Geometry: final body of the model. Coordinates: model frame, mm. Coordinates: 2 decimals unless noted, no trailing zeros. Order: outer loops, then holes, each group sorted by start corner. A loop starts at its lowest first (then second) coordinate and runs counter-clockwise, first axis right, second up. Notation, with made-up numbers: (-22, 60) -> (37, 60) arc R19 ccw to (37, 83) -> close; hole circle Ø3 at (72.5, -23.75). An arc over 180 degrees is marked (long way). Use one line per item in the form item = value.
Autodesk Inventor part; units mm, degrees
ref_plane "YZ Plane" through (0, 0, 0) normal (1, 0, 0) x (0, 1, 0)
ref_plane "XZ Plane" through (0, 0, 0) normal (0, 1, 0) x (-1, 0, 0)
ref_plane "XY Plane" through (0, 0, 0) normal (0, 0, 1) x (1, 0, 0)
sketch "Sketch1" plane through (0, 0, 0) normal (0, 0, 1) x (1, 0, 0)
  line L0 (0, 0) -> (50.8, 0) construction
  line L1 (50.8, 0) -> (50.8, 203.2) construction
  line L2 (50.8, 203.2) -> (0, 203.2) construction
  line L3 (0, 203.2) -> (0, 0) construction
  line L4 (-76.2, 0) -> (177.8, 0) construction
  line L5 (177.8, 0) -> (177.8, -76.2) construction
  line L6 (177.8, -76.2) -> (-76.2, -76.2) construction
  line L7 (-76.2, -76.2) -> (-76.2, 0) construction
  line L8 (165.1, -33.3375) -> (165.1, -68.2625) construction
  circle A0 centre (165.1, -33.3375) radius 4.7625 construction
  line L9 (174.625, -3.175) -> (-73.025, -3.175) construction
  line L10 (-73.025, -3.175) -> (-73.025, -73.025) construction
  line L11 (-73.025, -73.025) -> (174.625, -73.025) construction
  line L12 (174.625, -73.025) -> (174.625, -3.175) construction
  circle A1 centre (165.1, -68.2625) radius 4.7625 construction
  line L13 (-76.2, -76.2) -> (-76.2, 0)
  line L14 (-76.2, 0) -> (0, 101.6)
  line L15 (0, 101.6) -> (50.8, 101.6)
  line L16 (50.8, 101.6) -> (177.8, 0)
  line L17 (177.8, 0) -> (177.8, -76.2)
  line L18 (177.8, -76.2) -> (-76.2, -76.2)
  line L19 (50.8, 101.6) -> (50.8, 0) construction
  line L20 (50.8, 0) -> (177.8, 0) construction
  line L21 (0, 101.6) -> (0, 0) construction
  line L22 (0, 0) -> (-76.2, 0) construction
  line L23 (60.325, 9.525) -> (60.325, 77.7161) construction
  line L24 (50.8, 85.3361) -> (157.4701, 0)
  line L25 (145.5638, 9.525) -> (60.325, 9.525) construction
  line L26 (-60.325, 0) -> (0, 80.4333)
  line L27 (-9.525, 67.7333) -> (-9.525, 9.525) construction
  line L28 (-9.525, 9.525) -> (-53.1813, 9.525) construction
  line L29 (-60.325, 0) -> (0, 0)
  line L30 (0, 80.4333) -> (0, 0)
  line L31 (50.8, 85.3361) -> (50.8, 0)
  line L32 (50.8, 0) -> (157.4701, 0)
  line L33 (-9.525, 9.525) -> (-9.525, 0) construction
  line L34 (0, 4.7625) -> (50.8, 4.7625) construction
  line L35 (12.7, 34.925) -> (38.1, 34.925) construction
  line L36 (-6.35, 71.9667) -> (-6.35, 0)
  line L37 (57.15, 80.2561) -> (57.15, 0)
  point P0 (152.4, -50.8)
  point P1 (165.1, -50.8)
  point P2 (139.7, -68.2625)
  point P3 (139.7, -33.3375)
  point P4 (127, -50.8)
  point P5 (114.3, -68.2625)
  point P6 (114.3, -33.3375)
  point P7 (101.6, -50.8)
  point P8 (88.9, -68.2625)
  point P9 (88.9, -33.3375)
  point P10 (76.2, -50.8)
  point P11 (63.5, -68.2625)
  point P12 (63.5, -33.3375)
  point P13 (50.8, -50.8)
  point P14 (38.1, -68.2625)
  point P15 (38.1, -33.3375)
  point P16 (25.4, -50.8)
  point P17 (12.7, -68.2625)
  point P18 (12.7, -33.3375)
  point P19 (0, -50.8)
  point P20 (-12.7, -68.2625)
  point P21 (-12.7, -33.3375)
  point P22 (-25.4, -50.8)
  point P23 (-38.1, -68.2625)
  point P24 (-38.1, -33.3375)
  point P25 (-50.8, -50.8)
  point P26 (-63.5, -68.2625)
  point P27 (-63.5, -33.3375)
  point P28 (-76.2, -50.8)
  point P29 (12.7, 76.2)
  point P30 (38.1, 76.2)
  point P31 (-9.525, 4.7625)
  point P32 (25.4, 4.7625)
  point P33 (25.4, 34.925)
  dimension "d0" = 50.8
  dimension "d1" = 203.2
  dimension "d2" = 254
  dimension "d3" = 76.2
  dimension "d4" = 127
  dimension "d5" = 12.7
  dimension "d6" = 12.7
  dimension "d7" = 9.525
  dimension "d8" = 3.175
  dimension "d9" = 9.525
  dimension "d12" = 25.4
  dimension "d17" = 25.4
  dimension "d18" = 34.925
  dimension "d19" = 25.4
  dimension "d20" = 12.7
  dimension "d21" = 9.525
  dimension "d22" = 9.525
  dimension "d32" = 111.125
  dimension "d33" = 41.275
  dimension "d35" = 12.7
  dimension "d36" = 12.7
  dimension "d37" = 9.525
  dimension "d38" = 50.8
  dimension "d39" = 34.925
  dimension "d40" = 6.35
  dimension "d41" = 6.35
extrude "Extrusion1" add sketch "Sketch1" along normal blind 6.35 contours L13 L14 L15 L16 L17 L18 | L24 L37 L32 L31 | L26 L30 L29 L36
hole "Hole1" at (165.1, -33.3375, 0) at (165.1, -68.2625, 0) at (139.7, -68.2625, 0) at (139.7, -33.3375, 0) at (-38.1, -33.3375, 0) at (-63.5, -68.2625, 0) at (-63.5, -33.3375, 0) at (12.7, 76.2, 0) at (38.1, 76.2, 0) at (38.1, 34.925, 0) at (12.7, 34.925, 0) at (-38.1, -68.2625, 0) at (-12.7, -33.3375, 0) at (-12.7, -68.2625, 0) at (63.5, -33.3375, 0) at (63.5, -68.2625, 0) direction (0, 0, 1) diameter 3.9624 end through all
fillet "Fillet1" radius 6.604 12 edges at (50.8, 101.6, 3.175) (0, 101.6, 3.175) (177.8, 0, 3.175) (-76.2, 0, 3.175) (-76.2, -76.2, 3.175) (177.8, -76.2, 3.175) (-60.325, 0, 3.175) (157.4701, 0, 3.175) (-6.35, 0, 3.175) (57.15, 0, 3.175) (57.15, 80.2561, 3.175) (-6.35, 71.9667, 3.175)
sketch "Sketch2" plane through (0, 0, 6.35) normal (0, 0, 1) x (1, 0, 0)
  line L0 (0, -19.05) -> (50.8, -19.05)
  line L1 (50.8, -19.05) -> (50.8, -63.5)
  line L2 (50.8, -63.5) -> (0, -63.5)
  line L3 (0, -63.5) -> (0, -19.05)
  arc A0 (-6.35, 52.1547) -> (-18.2372, 56.1171) centre (-12.954, 52.1547) ccw
  line L4 (-18.2372, 56.1171) -> (-52.4002, 10.5664)
  arc A1 (-52.4002, 10.5664) -> (-47.117, 0) centre (-47.117, 6.604) ccw
  line L5 (-47.117, 0) -> (-12.954, 0)
  arc A2 (-12.954, 0) -> (-6.35, 6.604) centre (-12.954, 6.604) ccw
  line L6 (-6.35, 6.604) -> (-6.35, 52.1547)
  arc A3 (57.15, 6.604) -> (63.754, 0) centre (63.754, 6.604) ccw
  line L7 (63.754, 0) -> (138.6435, 0)
  arc A4 (138.6435, 0) -> (142.769, 11.7609) centre (138.6435, 6.604) ccw
  line L8 (142.769, 11.7609) -> (67.8795, 71.6725)
  arc A5 (67.8795, 71.6725) -> (57.15, 66.5156) centre (63.754, 66.5156) ccw
  line L9 (57.15, 66.5156) -> (57.15, 6.604)
  arc A6 (3.302, 101.6) -> (-1.9812, 98.9584) centre (3.302, 94.996) ccw
  line L10 (3.302, 101.6) -> (48.4834, 101.6)
  arc A7 (52.6089, 100.1529) -> (48.4834, 101.6) centre (48.4834, 94.996) ccw
  line L11 (52.6089, 100.1529) -> (175.3215, 1.9828)
  arc A8 (177.8, -3.174) -> (175.3215, 1.9828) centre (171.196, -3.174) ccw
  line L12 (177.8, -3.174) -> (177.8, -69.596)
  arc A9 (171.196, -76.2) -> (177.8, -69.596) centre (171.196, -69.596) ccw
  line L13 (171.196, -76.2) -> (-69.596, -76.2)
  arc A10 (-76.2, -69.596) -> (-69.596, -76.2) centre (-69.596, -69.596) ccw
  line L14 (-76.2, -69.596) -> (-76.2, -2.2013)
  arc A11 (-74.8792, 1.7611) -> (-76.2, -2.2013) centre (-69.596, -2.2013) ccw
  line L15 (-74.8792, 1.7611) -> (-1.9812, 98.9584)
  circle A12 centre (12.7, 34.925) radius 1.9812
  circle A13 centre (38.1, 76.2) radius 1.9812
  circle A14 centre (-63.5, -33.3375) radius 1.9812
  circle A15 centre (-38.1, -33.3375) radius 1.9812
  circle A16 centre (139.7, -68.2625) radius 1.9812
  circle A17 centre (165.1, -33.3375) radius 1.9812
  circle A18 centre (165.1, -68.2625) radius 1.9812
  circle A19 centre (139.7, -33.3375) radius 1.9812
  circle A20 centre (-63.5, -68.2625) radius 1.9812
  circle A21 centre (12.7, 76.2) radius 1.9812
  circle A22 centre (38.1, 34.925) radius 1.9812
  circle A23 centre (-38.1, -68.2625) radius 1.9812
  circle A24 centre (-12.7, -68.2625) radius 1.9812
  circle A25 centre (-12.7, -33.3375) radius 1.9812
  line L16 (76.2, -19.05) -> (127, -19.05)
  line L17 (127, -19.05) -> (127, -63.5)
  line L18 (127, -63.5) -> (76.2, -63.5)
  line L19 (76.2, -63.5) -> (76.2, -19.05)
  circle A26 centre (63.5, -33.3375) radius 1.9812
  circle A27 centre (63.5, -68.2625) radius 1.9812
  point P0 (0, 0)
  dimension "d44" = 12.7
  dimension "d45" = 19.05
  dimension "d49" = 12.7
  dimension "d52" = 12.7
  dimension "d53" = 12.7
  dimension "d54" = 12.7
extrude "Extrusion2" cut sketch "Sketch2" against normal blind 25.4 contours L0 L1 L2 L3 | L16 L17 L18 L19
fillet "Fillet2" radius 6.604 8 edges at (0, -63.5, 3.175) (0, -19.05, 3.175) (50.8, -63.5, 3.175) (50.8, -19.05, 3.175) (76.2, -63.5, 3.175) (76.2, -19.05, 3.175) (127, -19.05, 3.175) (127, -63.5, 3.175)
hole "Hole2" at (114.3, -33.3375, 0) at (101.6, -50.8, 0) at (88.9, -33.3375, 0) at (38.1, -33.3375, 0) at (25.4, -50.8, 0) at (12.7, -33.3375, 0) at (0, 4.7625, 0) at (50.8, 4.7625, 0) direction (0, 0, 1) diameter 5.1054 end through all
equation "\"d52\" = d51"
equation "\"d53\" = d49"
equation "\"d54\" = d53"
properties part number "EL2-S-002" material "Aluminum 6061"
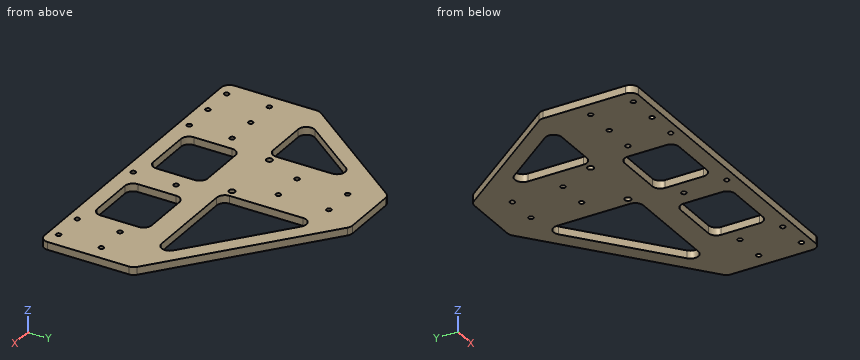
1) Contact query for a flat-ended pin moving along its axis: P1, Ø2, axis at y = 12.5, z = 2.5, coming from the -X side (3 decimals). Output: stop coordinate, or through.
Results found:
P1 = -67.575
2) Section A-A, the plane x = 29. Output: boundary loops of the cut face in (y, z), and give its area (3 significant figures).
Results found:
outline = (-76.2, 0) -> (-63.5, 0) -> (-63.5, 6.35) -> (-76.2, 6.35) -> close; (-19.05, 0) -> (101.6, 0) -> (101.6, 6.35) -> (-19.05, 6.35) -> close
area = 847 mm2
3) Section D-D, the plane y = 19.5. Output: boundary loops of the cut face in (x, z) (3 decimals).
Results found:
outline = (-61.575, 0) -> (-45.7, 0) -> (-45.7, 6.35) -> (-61.575, 6.35) -> close; (-6.35, 0) -> (57.15, 0) -> (57.15, 6.35) -> (-6.35, 6.35) -> close; (133.095, 0) -> (153.425, 0) -> (153.425, 6.35) -> (133.095, 6.35) -> close
4) Material intervals for probe 1 along X at (y, z) = (-45.5, 1.75); probe 2 along Y at (x, z) = (12.7, 3.5); probe 3 along Y at (x, z) = (32.5, 2.75), sorted ascending. Write a range as from..to.
Results found:
probe_1 = -76.2..0, 50.8..76.2, 127..177.8
probe_2 = -76.2..-63.5, -19.05..32.94, 36.91..74.22, 78.18..101.6
probe_3 = -76.2..-63.5, -19.05..101.6
5) Section C-C, the plane y = 69. Output: boundary loops of the cut face in (x, z).
Results found:
outline = (-24.45, 0) -> (57.64, 0) -> (57.64, 6.35) -> (-24.45, 6.35) -> close; (71.22, 0) -> (91.55, 0) -> (91.55, 6.35) -> (71.22, 6.35) -> close
6) Section B-B, the plane x = 80. Output: boundary loops of the cut face in (y, z), and give its area (3 significant figures).
Results found:
outline = (-76.2, 0) -> (-62.88, 0) -> (-62.88, 6.35) -> (-76.2, 6.35) -> close; (-19.67, 0) -> (0, 0) -> (0, 6.35) -> (-19.67, 6.35) -> close; (61.98, 0) -> (78.24, 0) -> (78.24, 6.35) -> (61.98, 6.35) -> close
area = 313 mm2
